CAD build for the part. Positions are in the model's coordinates, mm. A direction names the side the tool comes from. Give positions to 0.01 mm unless a question says otherwise; leave off trailing zeros. Order: outer loops, then holes, each group sorted by start corner. A loop starts at its lowest first (then second) coordinate and runs counter-clockwise, first axis right, second up.
Item 1: Flat gauge pins, fed straight in: P1, Ø22.5, axis at x = -30, y = -1, coming from the +Z side; P2, Ø5.5, axis at x = 45.11, y = 25.78, coming from the +Z side; P3, Ø17.5, axis at x = 46.5, z = 18, coming from the -Y side; P4, Ø1.5, axis at y = 8.5, z = 28.5, coming from the +X side. Where does each tip first touch, or does it go through?
Item 2: Two-plate mould, pull along Y, no slides. Class faces 4 (the cylindrical face through (14.95, -5.76, 14.22)), 5 (the flat face through (15.364, -30, 18)), 6 (the flat face through (-13, 37.719, 24)), 7 (the flat face through (-21, -37.719, 24)): released by +Y, released by -Y, zero draft, split by the parting line, or undercut.
Item 3: Band-saw the part on C-C on y = -26. Give the cut face in (x, z), plus the area to 3 significant figures.
Item 4: Which spindle directions (+Z, -Z, +X, -X, +Y, -Y) get a long thin tool onto all of the face, cutting with end or side? Do faces 1 (the flat face through (-34, -1, 9.722)), 2 (the flat face through (27, -21.332, 10)), 3 (the flat face through (-25, -10.159, 45)). Say none if no direction does.
Item 5: Wall check: L1, parallel to Y at x = -30, z = 43.5; L2, parallel to X at y = -5.5, z = 7; L3, parallel to Y at x = 19, z = 13. Give the ranges that are in metal, low to high.
Item 6: Band-saw the part on B-B on z = 11. Give the cut face in (x, y) (1 decimal), plus the area to 3 significant figures.
Item 7: Band-saw the part on A-A on x = -5. Give the cut face in (y, z).
Item 8: Band-saw the part on D-D on z = 31. Give the cut face in (x, y) (1 decimal), plus the area to 3 significant figures.
```python
from build123d import *

# Parameters (mm, degrees)
F1_DEPTH      = 37.718965
F2_W          = 42.4428796396
F2_H          = 16.3872130215
F3_DEPTH      = 48.2236520451
F4_W          = 20.3172173351
F4_H          = 6.184624848
F5_DEPTH      = 56.7568631301
F5_DEPTH_BACK = 57.8078979084
F6_R          = 4.7625
F7_DEPTH      = 48.2236520451


with BuildPart() as f1:
    # F0 (on Front) → F1 (new body, symmetric)
    with BuildSketch(Plane.XZ):
        Polygon((-10.5103449896, 0), (57.8068979084, 0), (0, 48.2226520451), (-56.7558631301, 48.2226520451), (-56.7558631301, 9.7220684111), (-10.5103449896, 9.7220684111), align=None)
    extrude(amount=F1_DEPTH, both=True)

    # F2 (on face) → F3 (cut, through all)
    with BuildSketch(Plane.XY.offset(48.2226520451)):
        with Locations((36.5854580887, -29.5253584892)):
            Rectangle(F2_W, F2_H)
    extrude(amount=-F3_DEPTH, mode=Mode.SUBTRACT)

    # F4 (on Right) → F5 (cut, two sides)
    with BuildSketch(Plane.YZ) as f5_sk:
        with Locations((0, 45.1303396211)):
            Rectangle(F4_W, F4_H)
    extrude(amount=-F5_DEPTH, mode=Mode.SUBTRACT)
    extrude(f5_sk.sketch, amount=F5_DEPTH_BACK, mode=Mode.SUBTRACT)

    # F6 (on face) → F7 (cut, through all)
    with BuildSketch(Plane.XY.offset(48.2226520451)):
        with Locations((45.1068979084, 25.781035)):
            Circle(F6_R)
        with Locations((19.7068979084, 25.781035)):
            Circle(F6_R)
        with Locations((19.7068979084, -5.968965)):
            Circle(F6_R)
        with Locations((45.1068979084, -5.968965)):
            Circle(F6_R)
    extrude(amount=-F7_DEPTH, mode=Mode.SUBTRACT)


solid = f1.part
```
The answers:
1. P1: stops at z = 48.22
1. P2: passes through
1. P3: stops at y = -21.33
1. P4: stops at x = 24.54
2. face 4: undercut
2. face 5: zero draft
2. face 6: released by +Y
2. face 7: released by -Y
3. outline: (-56.76, 9.72) - (-10.51, 9.72) - (-10.51, 0) - (15.36, 0) - (15.36, 35.41) - (0, 48.22) - (-56.76, 48.22) - close
3. area: 2,930 mm2
4. face 1: -Z, -X, +Y, -Y
4. face 2: +Z, -Z, +X, -Y
4. face 3: +Z, +X, -X
5. L1: y = -37.72 to -10.16, 10.16 to 37.72
5. L2: x = -10.51 to 14.97, 24.45 to 40.37
5. L3: y = -21.33 to -10.68, -1.26 to 21.07, 30.49 to 37.72
6. outline: (-56.8, -37.7) - (15.4, -37.7) - (15.4, -21.3) - (44.6, -21.3) - (44.6, -10.7) arc R4.8 cw to (44.6, -1.2) - (44.6, 21) arc R4.8 cw to (44.6, 30.5) - (44.6, 37.7) - (-56.8, 37.7) - close; hole circle Ø9.5 at (19.7, -6); hole circle Ø9.5 at (19.7, 25.8)
6. area: 6,960 mm2
7. outline: (-37.72, 0) - (37.72, 0) - (37.72, 48.22) - (10.16, 48.22) - (10.16, 42.04) - (-10.16, 42.04) - (-10.16, 48.22) - (-37.72, 48.22) - close
8. outline: (-56.8, -37.7) - (15.4, -37.7) - (15.4, -21.3) - (20.6, -21.3) - (20.6, -10.6) arc R4.8 cw (long way) to (20.6, -1.3) - (20.6, 21.1) arc R4.8 cw (long way) to (20.6, 30.5) - (20.6, 37.7) - (-56.8, 37.7) - close
8. area: 5,660 mm2
